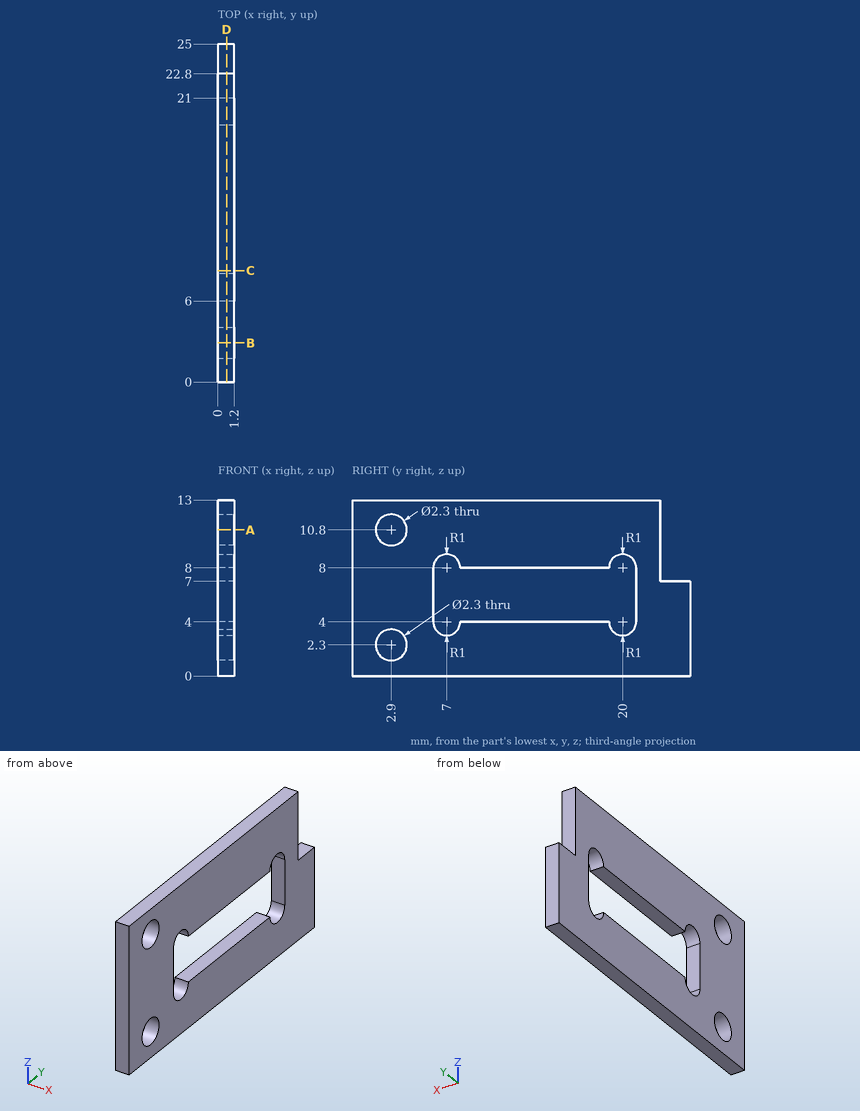
For this review, use the dimensioned drawing (mm, ordinates from the lowest corner) and the shaded views. Give positions to 0.01 mm unless a question says otherwise; leave off trailing zeros. Order: outer loops, then holes, each group sorted by start corner. A loop starts at its lowest first (then second) coordinate and runs counter-clockwise, first axis right, second up. Notation, with made-up numbers: (45.5, -35) - (52.5, -35) arc R18 ccw to (52.5, -3) - close; hole circle Ø9 at (85.25, -23.75). An arc over 180 degrees is marked (long way). Use a Markdown table: item, result. Add a question column.
(1) Add section A-A on z = 10.8. Give the boundary of the cut face in (x, y).
(2) Add section D-D on x = 0.65. Give the boundary of the cut face in (y, z).
(3) Add section C-C on y = 8.25. Give the boundary of the cut face in (x, z).
(4) Wall thickness on probe 1 along Z at (x, y) = (0.1, 3); probe 2 along Z at (x, y) = (0.6, 13); probe 3 along Y at (x, z) = (0.45, 2.3): over which ranges is each line inside the solid? List them lowest first. Write a range as [from, to].
(5) Add section B-B on y = 2.9. Give the boundary of the cut face in (x, z).
Report:
| question | item | result |
|---|---|---|
| 1 | outline | (0, 0) - (1.2, 0) - (1.2, 1.75) - (0, 1.75) - close; (0, 4.05) - (1.2, 4.05) - (1.2, 22.8) - (0, 22.8) - close |
| 2 | outline | (0, 0) - (25, 0) - (25, 7) - (22.8, 7) - (22.8, 13) - (0, 13) - close; hole circle Ø2.3 at (2.9, 2.3); hole circle Ø2.3 at (2.9, 10.8); hole (6, 4) arc R1 ccw to (8, 4) - (19, 4) arc R1 ccw to (21, 4) - (21, 8) arc R1 ccw to (19, 8) - (8, 8) arc R1 ccw to (6, 8) - close |
| 3 | outline | (0, 0) - (1.2, 0) - (1.2, 4) - (0, 4) - close; (0, 8) - (1.2, 8) - (1.2, 13) - (0, 13) - close |
| 4 | probe 1 | z = [0, 1.15], [3.45, 9.65], [11.95, 13] |
| 4 | probe 2 | z = [0, 4], [8, 13] |
| 4 | probe 3 | y = [0, 1.75], [4.05, 25] |
| 5 | outline | (0, 0) - (1.2, 0) - (1.2, 1.15) - (0, 1.15) - close; (0, 3.45) - (1.2, 3.45) - (1.2, 9.65) - (0, 9.65) - close; (0, 11.95) - (1.2, 11.95) - (1.2, 13) - (0, 13) - close |
